Model file for the job. Use its own axes, mm. Face numbers are marked on the shaded views. A direction names the side the tool comes from. Coordinates: 2 decimals unless noted, no trailing zeros. Write each loop counter-clockwise with the first axis right and the second up, starting at its lowest first coordinate (ties: lowest second). Pieces come first, ordered by that corner, then holes. Notation, with made-up numbers: M 79.5,-30 L 117.5,-30 A17 ccw 117.5,-3 Z; hole C 80,2 d6. An arc over 180 degrees is marked long. Use CSV: the item, a comma, the result in double quotes. Start each with the question number.
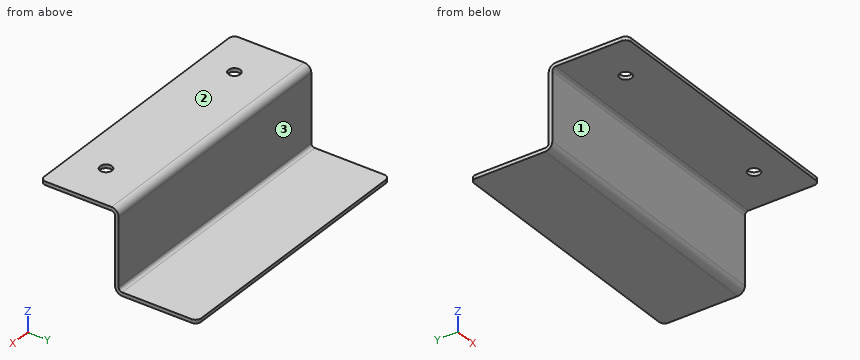
from build123d import *

# Parameters (mm, degrees)
BOSS_EXTRUDE1_DEPTH = 152.4
FILLET1_R           = 2.032
FILLET2_R           = 4.064
FILLET3_R           = 3.175
SKETCH2_R           = 3.3655
CUT_EXTRUDE1_DEPTH  = 47.482


with BuildPart() as part:
    # Sketch1 → Boss-Extrude1 (new body)
    with BuildSketch(Plane(origin=(0, 0, 0), x_dir=(0, 0, -1), z_dir=(1, 0, 0))):
        Polygon((0, 0), (0, -44.45), (-44.45, -44.45), (-44.45, -88.9), (-42.418, -88.9), (-42.418, -46.482), (2.032, -46.482), (2.032, 0), align=None)
    extrude(amount=BOSS_EXTRUDE1_DEPTH)

    # Fillet1
    fillet1_edges = [part.edges().sort_by_distance(p)[0] for p in [
        (76.2, -46.482, 42.418),
        (76.2, -44.45, 0),
    ]]
    fillet(fillet1_edges, radius=FILLET1_R)

    # Fillet2
    fillet2_edges = [part.edges().sort_by_distance(p)[0] for p in [
        (76.2, -46.482, -2.032),
        (76.2, -44.45, 44.45),
    ]]
    fillet(fillet2_edges, radius=FILLET2_R)

    # Fillet3
    fillet3_edges = [part.edges().sort_by_distance(p)[0] for p in [
        (0, 0, -1.016),
        (152.4, -88.9, 43.434),
        (152.4, 0, -1.016),
        (0, -88.9, 43.434),
    ]]
    fillet(fillet3_edges, radius=FILLET3_R)

    # Sketch2 → Cut-Extrude1 (cut, through all)
    with BuildSketch(Plane.XY.offset(44.45)):
        with Locations((25.4, -69.85)):
            Circle(SKETCH2_R)
        with Locations((127, -69.85)):
            Circle(SKETCH2_R)
    extrude(amount=-CUT_EXTRUDE1_DEPTH, mode=Mode.SUBTRACT)


solid = part.part
1) Drop flat-ended pins along their axis: P1, Ø7.5, axis at x = 25.4, y = -69.85, coming from the -Z side; P2, Ø19, axis at x = 49, z = 17.5, coming from the -Y side; P3, Ø4, axis at x = 45, z = 18, coming from the +Y side. Give the stop position or say it passes through.
2) Band-saw the part on B-B on x = 127. List the corners of the cut face in (y, z).
3) Tool access for the marked faces 1, 2 and 3: list every direction of +Z, -Z, +X, -X, +Y, -Y with a clear straight run to the whole face (end or side of a thin tool).
4) Band-saw the part on D-D on z = 4. List the corners of the cut face in (x, y), then the cut area to 3 significant figures.
5) Band-saw the part on A-A on y = -69.85. List the corners of the cut face in (x, z), then the cut area to 3 significant figures.
6) Wall check: L1, parallel to Y at x = 39, z = 25.5; L2, parallel to Z at x = 48, y = -7; L3, parallel to Z at x = 97.5, y = -67. Give the ranges that are in metal, low to high. Write a range as [from, to].
7) Band-saw the part on C-C on x = 60.5. List the corners of the cut face in (y, z).
Findings below:
1,P1,"stops at z = 42.42"
1,P2,"stops at y = -46.48"
1,P3,"stops at y = -44.45"
2,outline,"M -88.9,42.42 L -73.22,42.42 L -73.22,44.45 L -88.9,44.45 Z; M -66.48,42.42 L -48.51,42.42 A2.03 cw -46.48,40.39 L -46.48,2.03 A4.06 ccw -42.42,-2.03 L 0,-2.03 L 0,0 L -42.42,0 A2.03 cw -44.45,2.03 L -44.45,40.39 A4.06 ccw -48.51,44.45 L -66.48,44.45 Z"
3,face 1,"-Z, +X, -X, -Y"
3,face 2,"+Z, +X, -X, +Y, -Y"
3,face 3,"+Z, +X, -X, +Y"
4,outline,"M 0,-46.48 L 152.4,-46.48 L 152.4,-44.45 L 0,-44.45 Z"
4,area,"310 mm2"
5,outline,"M 0,42.42 L 22.03,42.42 L 22.03,44.45 L 0,44.45 Z; M 28.77,42.42 L 123.63,42.42 L 123.63,44.45 L 28.77,44.45 Z; M 130.37,42.42 L 152.4,42.42 L 152.4,44.45 L 130.37,44.45 Z"
5,area,"282 mm2"
6,L1,"y = [-46.48, -44.45]"
6,L2,"z = [-2.03, 0]"
6,L3,"z = [42.42, 44.45]"
7,outline,"M -88.9,42.42 L -48.51,42.42 A2.03 cw -46.48,40.39 L -46.48,2.03 A4.06 ccw -42.42,-2.03 L 0,-2.03 L 0,0 L -42.42,0 A2.03 cw -44.45,2.03 L -44.45,40.39 A4.06 ccw -48.51,44.45 L -88.9,44.45 Z"
